Autodesk Inventor part; units mm, degrees
ref_plane "YZ Plane" through (0, 0, 0) normal (1, 0, 0) x (0, 1, 0)
ref_plane "XZ Plane" through (0, 0, 0) normal (0, 1, 0) x (-1, 0, 0)
ref_plane "XY Plane" through (0, 0, 0) normal (0, 0, 1) x (1, 0, 0)
sketch "스케치1" plane through (0, 0, 0) normal (0, 1, 0) x (-1, 0, 0)
  line L0 (30, 50) -> (-30, 50)
  line L1 (-30, 50) -> (-30, -80)
  line L2 (-30, -80) -> (30, -80)
  line L3 (30, -80) -> (30, 50)
  point P0 (0, 0)
  dimension "d0" = 130
  dimension "d1" = 60
  dimension "d2" = 30
  dimension "d3" = 50
extrude "돌출1" add sketch "스케치1" along normal blind 3
sketch "스케치2" plane through (0, 3, 0) normal (0, 1, 0) x (1, 0, 0)
  line L0 (-30, 80) -> (-30, -50)
  line L1 (-10, 54) -> (-30, 54)
  line L2 (-30, 54) -> (-30, 28)
  line L3 (-30, 28) -> (-10, 28)
  line L4 (-10, 28) -> (-10, 54)
  line L5 (-10, 2) -> (-30, 2)
  line L6 (-30, 2) -> (-30, -24)
  line L7 (-30, -24) -> (-10, -24)
  line L8 (-10, -24) -> (-10, 2)
  line L9 (-30, -50) -> (30, -50)
  point P0 (0, 0)
  dimension "d6" = 26
  dimension "d7" = 26
  dimension "d8" = 26
  dimension "d9" = 26
  dimension "d10" = 20
extrude "돌출2" cut sketch "스케치2" against normal blind 10
equation "\"d7\" = d6"
equation "\"d8\" = d7"
equation "\"d9\" = d8"
properties part number "라즈베리파이_SMPS 격리판" material "PMMA 플라스틱"
For this review, take the finished solid that the model builds, in its own axes (mm). A direction names the side the tool comes from. Coordinates: 2 decimals unless noted, no trailing zeros. Order: outer loops, then holes, each group sorted by start corner. A loop starts at its lowest first (then second) coordinate and runs counter-clockwise, first axis right, second up. Notation, with made-up numbers: (21, 42) - (44, 42) arc R14 ccw to (44, 66) - close; hole circle Ø9 at (-5.5, 24.5). An arc over 180 degrees is marked (long way). Answer as CSV lines item,"result". Start each with the question number.
1) To check wall thickness, follow line 1 along Z through (x, y) = (-20, 2.45); line 2 along X through (y, z) = (2.7, -49.5). State the ranges of each line that lie inside material, in increasing order. Write a range as [from, to].
2) Machinability: for faces 5 (the flat face through (-20, 2, -2)), 6 (the flat face through (-30, 1, -67)), which of the approach directions +Z, -Z, +X, -X, +Y, -Y give a long, thin tool a straight path to every point of the face, cutting with its end or side? Answer none if there is none.
3) Add section A-A (y = 1.75). State the section outline as (x, z) points, then the cut area to 3 significant figures.
4) Insertion check: P1, Ø3, axis at x = 22, z = 12, coming from the -Y side; P2, Ø0.9, axis at y = 2, z = -34.5, coming from the -X side. Each pin has a flat end and moves straight along its axis. Give the tip position at first contact, or say it passes through.
5) Draft analysis for pull direction Z (two halves, no side actions). For faces 1 (the flat face through (0, 1, -80)), 2 (the flat face through (-20, 2, -28)), 3 (the flat face through (0, 1, 50)), 4 (the flat face through (-10, 2, -41)), state which applies: +Z half, -Z half, draft (parallel to the pull), parting line (faces both ways), or undercut.
6) Add section B-B (z = -32.5). State the section outline as (x, y) points.
Result:
1,line 1,"[-80, -54], [-28, -2], [24, 50]"
1,line 2,"[-10, 30]"
2,face 5,"-X, +Y, -Y"
2,face 6,"+Z, -Z, -X, +Y, -Y"
3,outline,"(-30, -80) - (30, -80) - (30, 50) - (-30, 50) - (-30, 24) - (-10, 24) - (-10, -2) - (-30, -2) - (-30, -28) - (-10, -28) - (-10, -54) - (-30, -54) - close"
3,area,"6,760 mm^2"
4,P1,"y = 0"
4,P2,"x = -10"
5,face 1,"-Z half"
5,face 2,"undercut"
5,face 3,"+Z half"
5,face 4,"undercut"
6,outline,"(-10, 0) - (30, 0) - (30, 3) - (-10, 3) - close"
